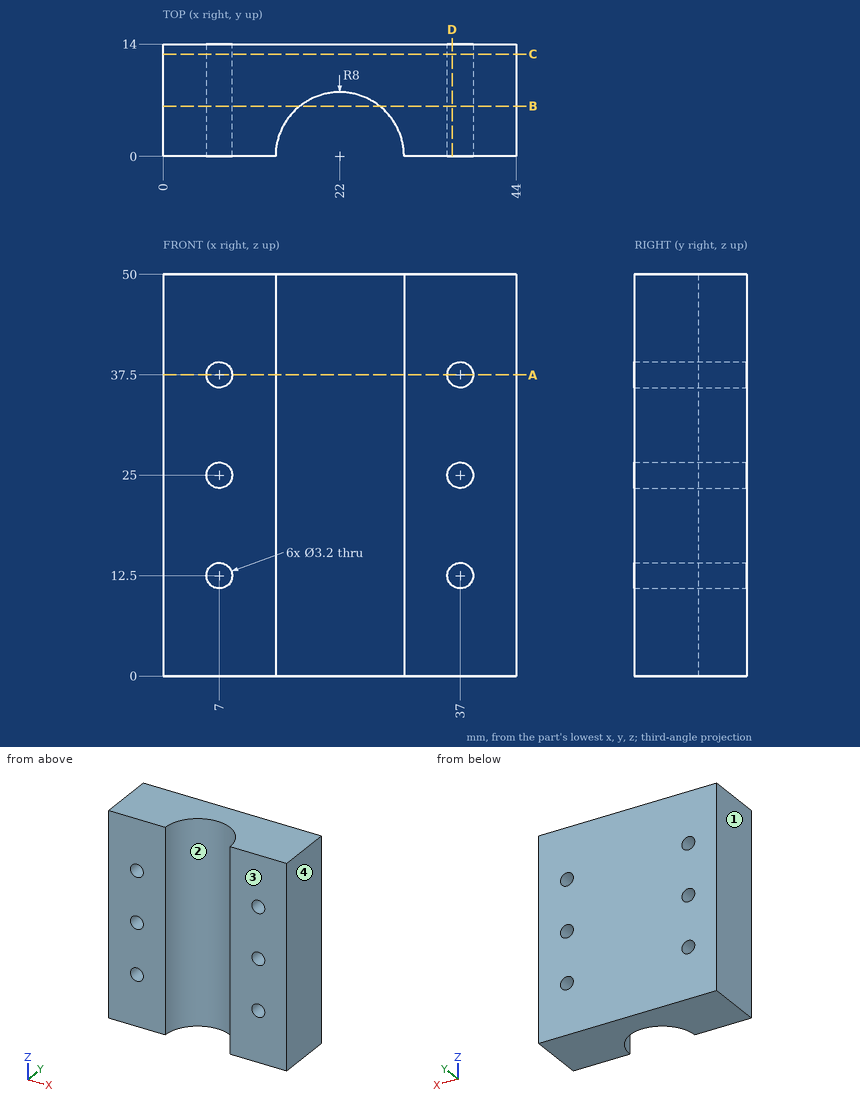
Source: three-view drawing plus pictorial views. Frame: mm from the lowest corner of the part. Give positions to 0.01 mm unless a question says otherwise; leave off trailing zeros. Loops run counter-clockwise (first coordinate to the right, second up) from the corner with the lowest first, then second, coordinate; pieces in that order, holes last. Notation, with made-up numbers: (-7.75, 26.5) -> (28.25, 26.5) arc R24 ccw to (28.25, 59.5) -> close; hole circle Ø7 at (21.5, 6.5). An arc over 180 degrees is marked (long way). Use a Markdown table: item, result. Add a question column.
(1) Ray query, line 1 (Z direction, x = 7, y = 11); line 2 (X direction, y = 5.75, z = 13); line 3 (Z direction, x = 6, y = 12). Return the intervals inside material, ascending.
(2) Pull-direction query (X, two-part tool) for the marked faces 1, 2, 3 and 4; classes: +X half, -X half, draft (parallel to the pull), parting line (faces both ways), or undercut.
(3) First-contact query: pin 1 Ø3 at (x, z) = (7, 37.5) entering from -Y. Flat tip, straight axial feed; report the tip coordinate or a pass-through.
(4) Section query B-B (y = 6.25). Output: boundary loops of the cut face in (x, z).
(5) Section query C-C (y = 12.75). Output: boundary loops of the cut face in (x, z).
(6) Section query A-A (z = 37.5). Output: boundary loops of the cut face in (x, y).
(7) Section query D-D (x = 36). Output: boundary loops of the cut face in (y, z), then the cut area to 3 significant figures.
Checked values:
| question | item | result |
|---|---|---|
| 1 | line 1 | 0 to 10.9, 14.1 to 23.4, 26.6 to 35.9, 39.1 to 50 |
| 1 | line 2 | 0 to 5.48, 8.52 to 16.44, 27.56 to 35.48, 38.52 to 44 |
| 1 | line 3 | 0 to 11.25, 13.75 to 23.75, 26.25 to 36.25, 38.75 to 50 |
| 2 | face 1 | -X half |
| 2 | face 2 | undercut |
| 2 | face 3 | draft |
| 2 | face 4 | +X half |
| 3 | pin 1 | through |
| 4 | outline | (0, 0) -> (17.01, 0) -> (17.01, 50) -> (0, 50) -> close; (26.99, 0) -> (44, 0) -> (44, 50) -> (26.99, 50) -> close; hole circle Ø3.2 at (7, 12.5); hole circle Ø3.2 at (7, 25); hole circle Ø3.2 at (7, 37.5); hole circle Ø3.2 at (37, 12.5); hole circle Ø3.2 at (37, 25); hole circle Ø3.2 at (37, 37.5) |
| 5 | outline | (0, 0) -> (44, 0) -> (44, 50) -> (0, 50) -> close; hole circle Ø3.2 at (7, 12.5); hole circle Ø3.2 at (7, 25); hole circle Ø3.2 at (7, 37.5); hole circle Ø3.2 at (37, 12.5); hole circle Ø3.2 at (37, 25); hole circle Ø3.2 at (37, 37.5) |
| 6 | outline | (0, 0) -> (5.4, 0) -> (5.4, 14) -> (0, 14) -> close; (8.6, 0) -> (14, 0) arc R8 cw to (30, 0) -> (35.4, 0) -> (35.4, 14) -> (8.6, 14) -> close; (38.6, 0) -> (44, 0) -> (44, 14) -> (38.6, 14) -> close |
| 7 | outline | (0, 0) -> (14, 0) -> (14, 11.25) -> (0, 11.25) -> close; (0, 13.75) -> (14, 13.75) -> (14, 23.75) -> (0, 23.75) -> close; (0, 26.25) -> (14, 26.25) -> (14, 36.25) -> (0, 36.25) -> close; (0, 38.75) -> (14, 38.75) -> (14, 50) -> (0, 50) -> close |
| 7 | area | 595 mm^2 |
